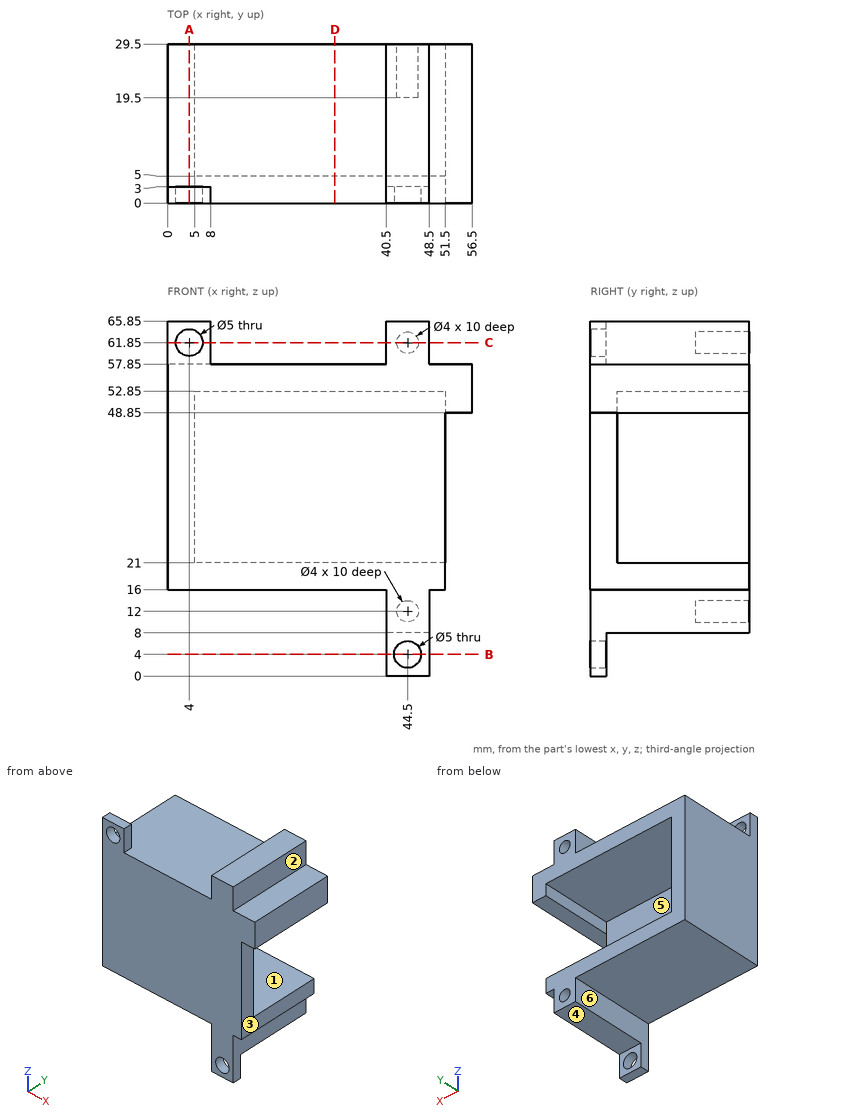
Geometry check sheet. Reference: drawing and pictorial views, mm from the part's lowest x, y, z. A direction names the side the tool comes from. Give positions to 0.01 mm unless a question says otherwise; leave off trailing zeros. Order: outer loops, then holes, each group sorted by start corner. A loop starts at its lowest first (then second) coordinate and runs counter-clockwise, first axis right, second up. Notation, with made-up numbers: M 76.25,77.25 L 101.25,77.25 A25 ccw 101.25,105.25 Z; hole C 67,34 d10. An arc over 180 degrees is marked long. Return JSON: item names as keys, results as strings. Group by question number.
1) Section check B-B on z = 4. Record the cut outline in (x, y).
2) Scan lines: line 1 (X direction, y = 1.45, z = 61.85); line 2 (X direction, y = 22.75, z = 12); line 3 (Z direction, x = 44.5, y = 1.5). Record each from-to range of solid material in increasing order.
3) Section check A-A on x = 4. Record the cut outline in (y, z).
4) Section check D-D on x = 31. Record the cut outline in (y, z), and give its area (3 significant figures).
5) Access from +Z, -Z, +X, -X, +Y, -Y to the whole of each face (thin tool, end or side, straight path). Record for the marked faces 1, 2 and 3.
6) Mould release check, pull along Z, two halves, no side actions. Record for the marked faces 4, 5 and 6: pulls with the +Z half, pulls with the -Z half, needs draft (parallel to the pull), parting line crosses it, or undercut.
7) Go/stop test with flat-tipped pins: pin 1 Ø13 at (y, z) = (21.5, 10.5) entering from +X; pin 2 Ø5 at (x, y) = (28, 15.5) entering from +Z; pin 3 Ø3 at (x, y) = (13.5, 7.5) entering from -Z; pin 4 Ø4.5 at (y, z) = (13, 50.5) entering from -X. Record where each tip stops, or that it passes through.
8) Section check C-C on z = 61.85. Record the cut outline in (x, y), and give its area (3 significant figures).
Answer block:
{
 "1": {"outline": "M 40.5,0 L 42,0 L 42,3 L 40.5,3 Z; M 47,0 L 48.5,0 L 48.5,3 L 47,3 Z"},
 "2": {"line 1": "x = 0 to 1.5, 6.5 to 8, 40.5 to 48.5", "line 2": "x = 40.5 to 42.5, 46.5 to 48.5", "line 3": "z = 0 to 1.5, 6.5 to 65.85"},
 "3": {"outline": "M 0,16 L 29.5,16 L 29.5,57.85 L 3,57.85 L 3,59.35 L 0,59.35 Z; M 0,64.35 L 3,64.35 L 3,65.85 L 0,65.85 Z"},
 "4": {"outline": "M 0,16 L 29.5,16 L 29.5,21 L 5,21 L 5,52.85 L 29.5,52.85 L 29.5,57.85 L 0,57.85 Z", "area": "454 mm^2"},
 "5": {"face 1": "+X, +Y", "face 2": "+Z, +X, +Y, -Y", "face 3": "-Z, +X, +Y, -Y"},
 "6": {"face 4": "pulls with the -Z half", "face 5": "undercut", "face 6": "needs draft"},
 "7": {"pin 1": "stops at x = 51.5", "pin 2": "stops at z = 57.85", "pin 3": "stops at z = 16", "pin 4": "stops at x = 0"},
 "8": {"outline": "M 0,0 L 1.5,0 L 1.5,3 L 0,3 Z; M 6.5,0 L 8,0 L 8,3 L 6.5,3 Z; M 40.5,0 L 48.5,0 L 48.5,29.5 L 46.5,29.5 L 46.5,19.5 L 42.5,19.5 L 42.5,29.5 L 40.5,29.5 Z", "area": "205 mm^2"}
}
